from build123d import *

# Parameters (mm, degrees)
F0_W     = 37.6
F0_H     = 28
F0_W_2   = 15
F0_H_2   = 26
F0_W_3   = 30
F1_DEPTH = 42
F2_W     = 30
F2_H     = 15
F2_W_2   = 60
F2_H_2   = 27
F3_DEPTH = 87.001
F4_W     = 61
F4_H     = 27
F5_DEPTH = 120.001


with BuildPart() as f1:
    # F0 (on Top) → F1 (new body)
    with BuildSketch(Plane.XY):
        Polygon((-373.474174, 103.589958), (-373.474174, 42.589958), (-358.974174, 42.589958), (-341.724174, 59.839958), (-324.474174, 42.589958), (-253.474174, 42.589958), (-253.474174, 129.589958), (-277.1233, 129.589958), (-277.1233, 122.589958), (-293.1233, 122.589958), (-293.1233, 129.589958), (-313.474174, 129.589958), (-313.474174, 103.589958), (-328.474174, 103.589958), (-358.474174, 103.589958), align=None)
        with Locations((-285.274174, 83.589958)):
            Rectangle(F0_W, F0_H, mode=Mode.SUBTRACT)
        with Locations((-365.974174, 116.589958)):
            Rectangle(F0_W_2, F0_H_2)
        with Locations((-343.474174, 116.589958)):
            Rectangle(F0_W_3, F0_H_2)
        with Locations((-320.974174, 116.589958)):
            Rectangle(F0_W_2, F0_H_2)
    extrude(amount=F1_DEPTH)

    # F2 (on face) → F3 (cut, through all)
    with BuildSketch(Plane.XZ.offset(-42.589958)):
        with Locations((-343.474174, 34.5)):
            Rectangle(F2_W, F2_H)
        with Locations((-283.474174, 28.5)):
            Rectangle(F2_W_2, F2_H_2)
    extrude(amount=-F3_DEPTH, mode=Mode.SUBTRACT)

    # F4 (on face) → F5 (cut, through all)
    with BuildSketch(Plane.YZ.offset(-253.474174)):
        with Locations((73.089958, 28.5)):
            Rectangle(F4_W, F4_H)
    extrude(amount=-F5_DEPTH, mode=Mode.SUBTRACT)


solid = f1.part
Model file for the job. Use its own axes, mm. A direction names the side the tool comes from. Coordinates: 2 decimals unless noted, no trailing zeros. Order: outer loops, then holes, each group sorted by start corner. A loop starts at its lowest first (then second) coordinate and runs counter-clockwise, first axis right, second up. Notation, with made-up numbers: (7.25, 64.5) -> (30.25, 64.5) arc R14 ccw to (30.25, 82.5) -> close; hole circle Ø3 at (-38.75, 79.5). An arc over 180 degrees is marked (long way). Return JSON: item names as keys, results as strings. Group by question number.
Item 1: Saw through at A-A on x = -289. Write the cut outline in (y, z), then the cut area to 3 significant figures.
Item 2: Saw through at C-C on y = 118.5. Write the cut outline in (x, z).
Item 3: Tool access for faces 5 (the flat face through (-350.47, 51.094, 7.395)), 6 (the flat face through (-266.474, 83, 7)), 7 (the flat face through (-366, 117, 42)), 8 (the flat face through (-314, 87, 0)), 9 (the flat face through (-277.123, 126, 7)): list every direction of +Z, -Z, +X, -X, +Y, -Y with a clear straight run to the whole face (end or side of a thin tool).
Item 4: Pull direction X, two halves, no side cores. Call faces 1 (the flat face through (-373.474, 96, 11)), 2 (the flat face through (-286, 97.59, 7)), 3 (the flat face through (-358.474, 116, 34)), 4 (the flat face through (-343, 103.59, 25)): pulls with the +X half, pulls with the -X half, needs draft (parallel to the pull), parting line crosses it, or undercut.
Item 5: Saw through at B-B on z = 38.5. Write the cut outline in (x, y), then the cut area to 3 significant figures.
Item 6: Wall check: line 1 along X through (y, z) = (85, 6.5); line 2 along X through (y, z) = (110.5, 36); line 3 along Z through (x, y) = (-299, 64.5). Give the ranges that are in metal, low to high. Write a range as [from, to].
Item 7: Saw through at D-D on z = 3. Write the cut outline in (x, y).
Item 8: Flat gauge pins, fed straight in: P1, Ø4.5, axis at y = 115.5, z = 33.5, coming from the +X side; P2, Ø4, axis at y = 100.5, z = 33, coming from the -X side. Where does each tip first touch, or does it go through?
Values found:
{
 "1": {"outline": "(42.59, 0) -> (69.59, 0) -> (69.59, 15) -> (42.59, 15) -> close; (97.59, 0) -> (122.59, 0) -> (122.59, 15) -> (97.59, 15) -> close", "area": "780 mm2"},
 "2": {"outline": "(-373.47, 0) -> (-253.47, 0) -> (-253.47, 15) -> (-313.47, 15) -> (-313.47, 42) -> (-328.47, 42) -> (-328.47, 27) -> (-358.47, 27) -> (-358.47, 42) -> (-373.47, 42) -> close"},
 "3": {"face 5": "+Z, -Z, -Y", "face 6": "+Z, -Z", "face 7": "+Z, +X, -X, +Y, -Y", "face 8": "-Z, +X, -X, +Y, -Y", "face 9": "+Z, -Z, +Y"},
 "4": {"face 1": "pulls with the -X half", "face 2": "undercut", "face 3": "undercut", "face 4": "needs draft"},
 "5": {"outline": "(-373.47, 103.59) -> (-358.47, 103.59) -> (-358.47, 129.59) -> (-373.47, 129.59) -> close; (-328.47, 103.59) -> (-313.47, 103.59) -> (-313.47, 129.59) -> (-328.47, 129.59) -> close", "area": "780 mm2"},
 "6": {"line 1": "x = [-373.47, -304.07], [-266.47, -253.47]", "line 2": "x = [-373.47, -358.47], [-328.47, -313.47]", "line 3": "z = [0, 15]"},
 "7": {"outline": "(-373.47, 42.59) -> (-358.97, 42.59) -> (-341.72, 59.84) -> (-324.47, 42.59) -> (-253.47, 42.59) -> (-253.47, 129.59) -> (-277.12, 129.59) -> (-277.12, 122.59) -> (-293.12, 122.59) -> (-293.12, 129.59) -> (-373.47, 129.59) -> close; hole (-304.07, 69.59) -> (-266.47, 69.59) -> (-266.47, 97.59) -> (-304.07, 97.59) -> close"},
 "8": {"P1": "stops at x = -313.47", "P2": "passes through"}
}
